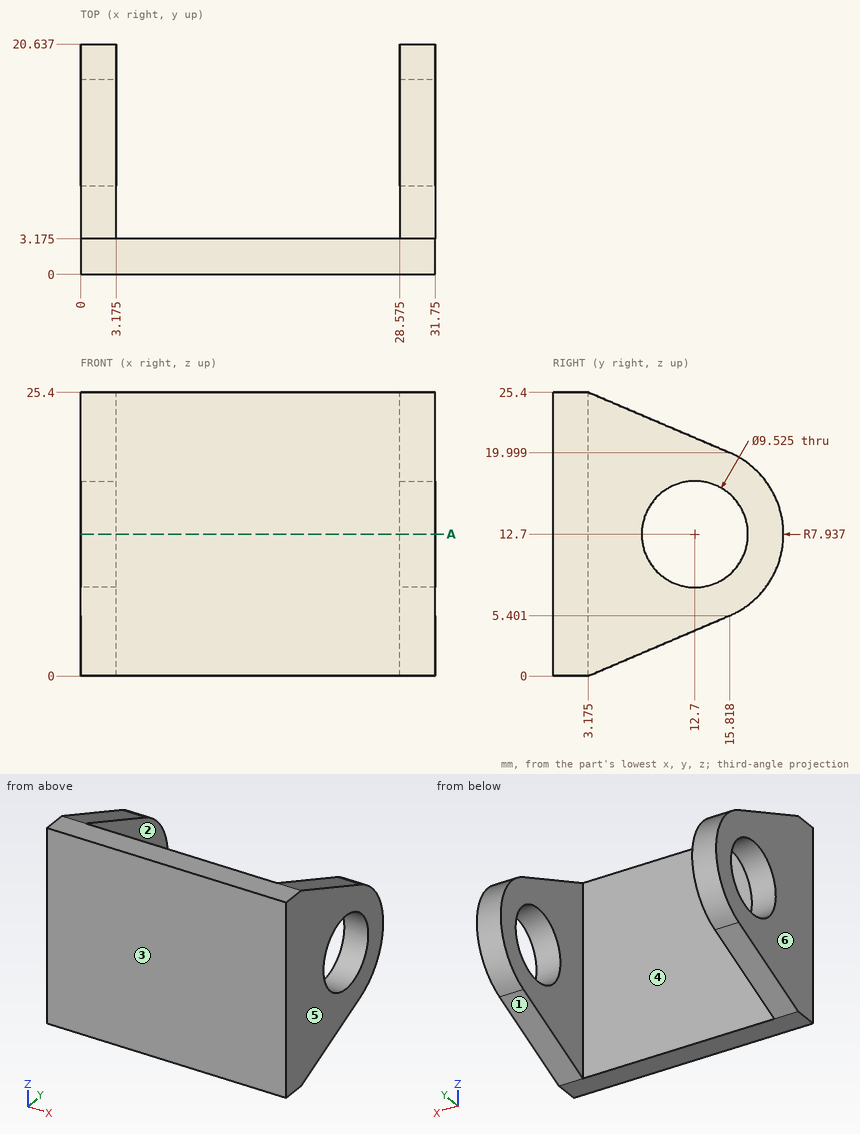
Design review of the part shown in the three views and the two pictorial views. Dimensions are in mm from the part's minimum x, y and z. A direction names the side the tool comes from. Give positions to 0.01 mm unless a question says otherwise; leave off trailing zeros. Put each result on its own line as item: value. Start each with the question number.
1. Mouldability with a two-part tool opening along X and no side actions: class the marked faces 3, 4, 5 and 6 as released by +X, released by -X, zero draft, split by the parting line, or undercut.
2. Wall thickness on probe 1 along Y at (x, z) = (12, 14) (1 decimal); probe 2 along Y at (x, z) = (2.5, 13.75) (1 decimal); probe 3 along Y at (x, z) = (29, 15) (1 decimal): over which ranges is each line inside the solid? List them lowest first.
3. Clearance check with flat-ended pins moving along their axes: P1, Ø1, axis at y = 15, z = 21, coming from the +X side (3 decimals); P2, Ø4, axis at x = 18.5, z = 4.5, coming from the +Y side (3 decimals). State where each tip first meets the part, or that it passes through.
4. For the marked faces 1 and 2, list the 3-axis set-ups (+Z, -Z, +X, -X, +Y, -Y) from which the entire face can be reached by the end or side of a thin tool; tool diameter is ignored.
5. We need section A-A on z = 12.7. State how many separate pieces and enclosed holes the cut face has, then the cut area to 3 significant figures.
Determined:
1. face 3: zero draft
1. face 4: undercut
1. face 5: released by +X
1. face 6: released by -X
2. probe 1: 0 to 3.2
2. probe 2: 0 to 8.1, 17.3 to 20.6
2. probe 3: 0 to 8.5, 16.9 to 20.3
3. P1: through
3. P2: y = 3.175
4. face 1: -Z, +X, -X, +Y
4. face 2: +Z, -Z, +Y
5. separate pieces: 3
5. enclosed holes: 0
5. area: 151 mm^2
